Geometry: see drawing. Coordinates: mm, zero at the bounding-box minimum. A direction names the side the tool comes from. Give positions to 0.01 mm unless a question says otherwise; leave off trailing zeros. Use one line per item in the form item = value.
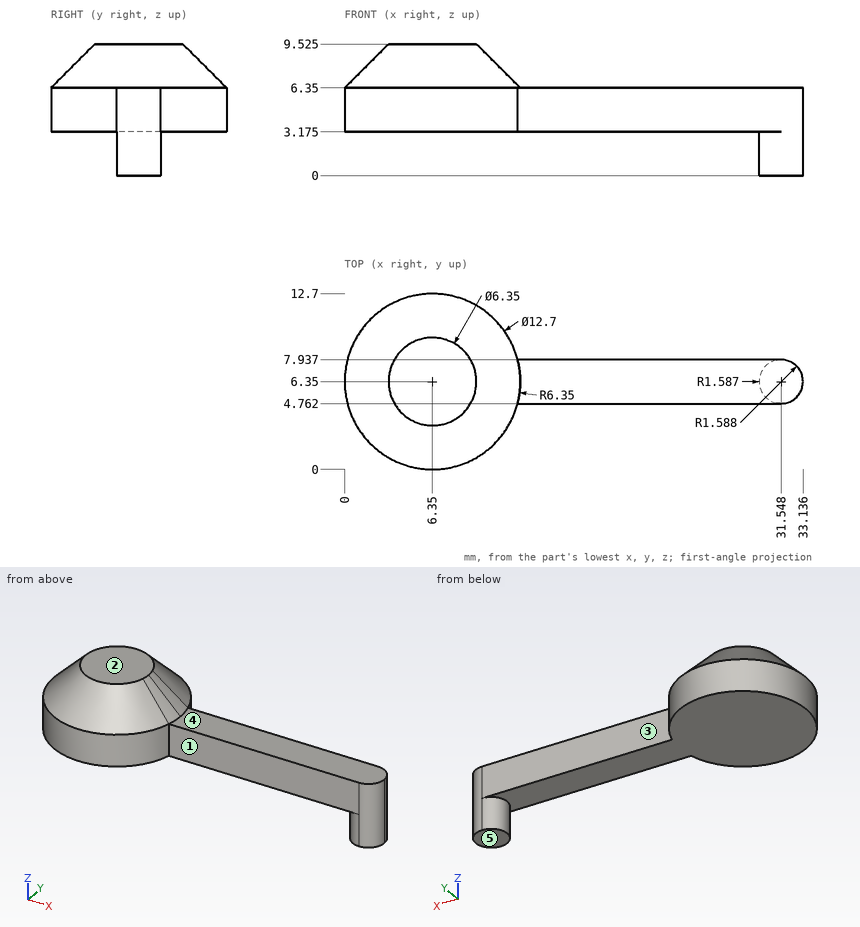
(1) Pin query (flat end, axial travel): P1, Ø3, axis at x = 10.5, y = 5, coming from the +Z side (1 decimal); P2, Ø4, axis at y = 3, z = 5, coming from the -X side (1 decimal); P3, Ø6.5, axis at x = 21, y = 6, coming from the -Z side (1 decimal); P4, Ø1.5, axis at x = 23, y = 6.5, coming from the +Z side. Return the tip coordinate at first contact, or that it passes through.
Solution:
P1 = 9.5
P2 = 0.1
P3 = 3.2
P4 = 6.35
(2) Access query for the marked faces 1, 2, 3, 4 and 5. Directions: +Z, -Z, +X, -X, +Y, -Y. A direction counts if a zero-diameter tool reaches every point of the face in a straight line with its end or side. Return the directions, or none.
Solution:
face_1 = +Z, -Z, +X, -Y
face_2 = +Z, +X, -X, +Y, -Y
face_3 = +Z, -Z, +X, +Y
face_4 = +Z, +X, +Y, -Y
face_5 = -Z, +X, -X, +Y, -Y
(3) Material intervals for L1, parallel to Y at x = 25, z = 4.25; L2, parallel to X at y = 6.25, z = 2.75 (1 decimal); L3, parallel to Z at x = 7, y = 8 (1 decimal), sorted ascending. Write a range as from..to.
Solution:
L1 = 4.76..7.94
L2 = 30..33.1
L3 = 3.2..9.5
